```python
from build123d import *

# Parameters (mm, degrees)
SKETCH2_W               = 42
SKETCH2_H               = 42
BOSS_EXTRUDE1_DEPTH     = 3
BOSS_EXTRUDE9_START     = 3
SKETCH2_5_W             = 5
SKETCH2_5_H             = 5
BOSS_EXTRUDE9_DEPTH     = 6
CUT_EXTRUDE3_DEPTH      = 32.032241298
CUT_EXTRUDE3_DEPTH_BACK = 32.032241298
SKETCH2_7_R             = 2
BOSS_EXTRUDE10_START    = -4
SKETCH2_6_W             = 5
SKETCH2_6_H             = 5
SKETCH2_6_R             = 2
BOSS_EXTRUDE10_DEPTH    = 4


with BuildPart() as part:
    # Sketch2 → Boss-Extrude1 (new body)
    with BuildSketch(Plane.XY):
        Rectangle(SKETCH2_W, SKETCH2_H)
    extrude(amount=BOSS_EXTRUDE1_DEPTH)

    # Sketch2<5> → Boss-Extrude9 (add)
    with BuildSketch(Plane.XY.offset(BOSS_EXTRUDE9_START)):
        with Locations((-15.5, 15.5)):
            Rectangle(SKETCH2_5_W, SKETCH2_5_H)
        with Locations((15.5, 15.5)):
            Rectangle(SKETCH2_5_W, SKETCH2_5_H)
        with Locations((15.5, -15.5)):
            Rectangle(SKETCH2_5_W, SKETCH2_5_H)
        with Locations((-15.5, -15.5)):
            Rectangle(SKETCH2_5_W, SKETCH2_5_H)
    extrude(amount=BOSS_EXTRUDE9_DEPTH)

    # Sketch2<7> → Cut-Extrude3 (cut, two sides: drawn at the far end of the back side and taken through both)
    with BuildSketch(Plane.XY.offset(-CUT_EXTRUDE3_DEPTH_BACK)):
        with Locations(Location((-15.5, 15.5, 0), (0, 0, 180))):
            Circle(SKETCH2_7_R)
        with Locations(Location((15.5, 15.5, 0), (0, 0, 180))):
            Circle(SKETCH2_7_R)
        with Locations(Location((15.5, -15.5, 0), (0, 0, 180))):
            Circle(SKETCH2_7_R)
        with Locations(Location((-15.5, -15.5, 0), (0, 0, 180))):
            Circle(SKETCH2_7_R)
    extrude(amount=CUT_EXTRUDE3_DEPTH + CUT_EXTRUDE3_DEPTH_BACK, mode=Mode.SUBTRACT)

    # Sketch2<6> → Boss-Extrude10 (add)
    # profile 1 of 4: a face of its own
    with BuildSketch(Plane.XY.offset(BOSS_EXTRUDE10_START)):
        with Locations((-15.5, -15.5)):
            Rectangle(SKETCH2_6_W, SKETCH2_6_H)
        with Locations(Location((-15.5, -15.5, 0), (0, 0, 180))):
            Circle(SKETCH2_6_R, mode=Mode.SUBTRACT)
    # profile 2 of 4: a face of its own
    with BuildSketch(Plane.XY.offset(BOSS_EXTRUDE10_START)):
        with Locations((15.5, -15.5)):
            Rectangle(SKETCH2_6_W, SKETCH2_6_H)
        with Locations(Location((15.5, -15.5, 0), (0, 0, 180))):
            Circle(SKETCH2_6_R, mode=Mode.SUBTRACT)
    # profile 3 of 4: a face of its own
    with BuildSketch(Plane.XY.offset(BOSS_EXTRUDE10_START)):
        with Locations((15.5, 15.5)):
            Rectangle(SKETCH2_6_W, SKETCH2_6_H)
        with Locations(Location((15.5, 15.5, 0), (0, 0, 180))):
            Circle(SKETCH2_6_R, mode=Mode.SUBTRACT)
    # profile 4 of 4: a face of its own
    with BuildSketch(Plane.XY.offset(BOSS_EXTRUDE10_START)):
        with Locations((-15.5, 15.5)):
            Rectangle(SKETCH2_6_W, SKETCH2_6_H)
        with Locations(Location((-15.5, 15.5, 0), (0, 0, 180))):
            Circle(SKETCH2_6_R, mode=Mode.SUBTRACT)
    extrude(amount=BOSS_EXTRUDE10_DEPTH)


solid = part.part
```
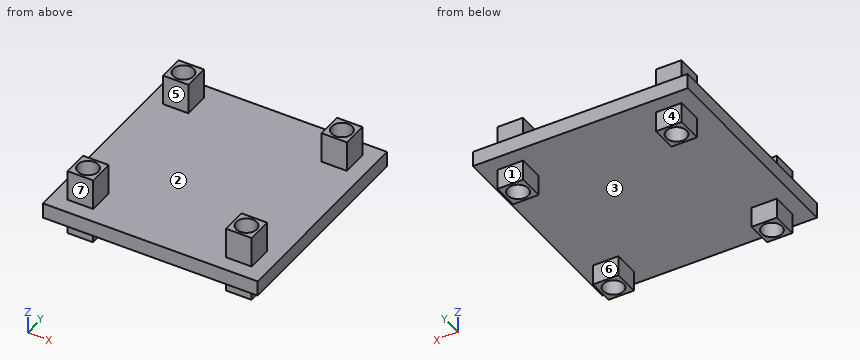
Here's how the part is built. I have some questions about the finished solid (model axes, mm). Face numbers are marked on the shaded views. A direction names the side the tool comes from. Round coordinates to 2 decimals unless told otherwise and drop trailing zeros. Write each loop counter-clockwise with the first axis right and the second up, starting at its lowest first coordinate (ties: lowest second). Pieces come first, ordered by that corner, then holes.
Q1. Please list where these lines run through material, in increasing order: probe 1 along Y at (x, z) = (15.5, -0.25); probe 2 along X at (y, z) = (15.5, 1.5).
Q2. If we section it at A-A on z = 6.5: Write out the boundary of the cut face in (x, y), plus the area to 3 significant figures.
Q3. If we section it at D-D on z = 2: Write out the boundary of the cut face in (x, y), plus the area to 3 significant figures.
Q4. If we section it at B-B on x = -15.5: Write out the boundary of the cut face in (y, z).
Q5. Will these pins go through, and if not, where does the flat tip stop? P1, Ø2, axis at x = 16.5, z = -3, coming from the -Y side; P2, Ø4, axis at y = -16, z = 5.5, coming from the +X side; P3, Ø3.5, axis at x = 15.5, y = 15.5, coming from the -Z side; P4, Ø3, axis at x = 8.5, y = 7, coming from the +Z side.
Q6. Which directions (+Z, -Z, +X, -X, +Y, -Y) give clear straight access to the entire face, cutting with the end or side of a thin tool? Please do the marked faces 4, 5, 6 and 7.
Q7. If we mould it in two halves opening along X, with no side actions, what happens to the marked faces 1, 2 and 3? For each: +X half, -X half, draft (parallel to the pull), parting line (faces both ways), or undercut.
Answer below:
1. probe 1: y = -18 to -17.5, -13.5 to -13, 13 to 13.5, 17.5 to 18
1. probe 2: x = -21 to -17.5, -13.5 to 13.5, 17.5 to 21
2. outline: (-18, -18) - (-13, -18) - (-13, -13) - (-18, -13) - close; (-18, 13) - (-13, 13) - (-13, 18) - (-18, 18) - close; (13, -18) - (18, -18) - (18, -13) - (13, -13) - close; (13, 13) - (18, 13) - (18, 18) - (13, 18) - close; hole circle Ø4 at (-15.5, -15.5); hole circle Ø4 at (-15.5, 15.5); hole circle Ø4 at (15.5, -15.5); hole circle Ø4 at (15.5, 15.5)
2. area: 49.7 mm2
3. outline: (-21, -21) - (21, -21) - (21, 21) - (-21, 21) - close; hole circle Ø4 at (-15.5, -15.5); hole circle Ø4 at (-15.5, 15.5); hole circle Ø4 at (15.5, -15.5); hole circle Ø4 at (15.5, 15.5)
3. area: 1,710 mm2
4. outline: (-21, 0) - (-18, 0) - (-18, -4) - (-17.5, -4) - (-17.5, 9) - (-18, 9) - (-18, 3) - (-21, 3) - close; (-13.5, -4) - (-13, -4) - (-13, 0) - (13, 0) - (13, -4) - (13.5, -4) - (13.5, 9) - (13, 9) - (13, 3) - (-13, 3) - (-13, 9) - (-13.5, 9) - close; (17.5, -4) - (18, -4) - (18, 0) - (21, 0) - (21, 3) - (18, 3) - (18, 9) - (17.5, 9) - close
5. P1: stops at y = -18
5. P2: stops at x = 18
5. P3: passes through
5. P4: stops at z = 3
6. face 4: -Z, +X, -X, +Y
6. face 5: +Z, +X, -X
6. face 6: -Z, +X, -X
6. face 7: +Z, +X, -X, -Y
7. face 1: draft
7. face 2: undercut
7. face 3: undercut
